```python
from build123d import *

# Parameters (mm, degrees)
SKETCH1_W                      = 88.6
SKETCH1_H                      = 58.4
BOSS_EXTRUDE1_DEPTH            = 1.6
F_2_7_2_7_DIAMETER_HOLE1_D     = 2.7
F_2_7_2_7_DIAMETER_HOLE1_DEPTH = 5.1
F_2_7_2_7_DIAMETER_HOLE1_TIP   = 0.811161836
LPATTERN1_COUNT                = 20
LPATTERN1_PITCH                = 2.54
LPATTERN1_COUNT_DIR2           = 2
LPATTERN1_PITCH_DIR2           = 2.54


with BuildPart() as part:
    # Sketch1 → Boss-Extrude1 (new body)
    with BuildSketch(Plane(origin=(0, 0, 0), x_dir=(1, 0, 0), z_dir=(0, 1, 0))):
        with Locations((11.8, 25.7)):
            Rectangle(SKETCH1_W, SKETCH1_H)
    extrude(amount=BOSS_EXTRUDE1_DEPTH)

    # Ø2.7 (2.7) Diameter Hole1
    with Locations(Plane(origin=(-29, 1.6, -49), x_dir=(0, 0, 1), z_dir=(0, 1, 0))):
        with Locations((0, 0), (0, 58), (49, 58), (49, 0)):
            Hole(F_2_7_2_7_DIAMETER_HOLE1_D / 2, depth=F_2_7_2_7_DIAMETER_HOLE1_DEPTH)
            with Locations((0, 0, -(F_2_7_2_7_DIAMETER_HOLE1_DEPTH + F_2_7_2_7_DIAMETER_HOLE1_TIP / 2))):  # 118° drill point
                Cone(0, F_2_7_2_7_DIAMETER_HOLE1_D / 2, F_2_7_2_7_DIAMETER_HOLE1_TIP, mode=Mode.SUBTRACT)

    # Sketch3 → Ø1.05 (1.05) Diameter Hole1 (revolve, cut)
    with BuildSketch(Plane(origin=(-24.13, 1.6, 1.27), x_dir=(0, 0, 1), z_dir=(1, 0, 0))):
        Polygon((0, 0), (0, 5.415451825), (0.525, 5.1), (0.525, 0), align=None)
    f_1_05_1_05_diameter_hole1 = revolve(axis=Axis((-24.13, 7.95, 1.27), (0, -1, 0)), mode=Mode.SUBTRACT)

    # LPattern1: 1.05 _1.05_ Diameter Hole1 20 × 2
    with Locations(*[(i * LPATTERN1_PITCH, 0, -j * LPATTERN1_PITCH_DIR2) for i in range(LPATTERN1_COUNT) for j in range(LPATTERN1_COUNT_DIR2) if (i, j) != (0, 0)]):
        add(f_1_05_1_05_diameter_hole1, mode=Mode.SUBTRACT)


solid = part.part
```
Work out the finished part from the listing and answer in its coordinate system (mm). Give positions to 0.01 mm unless a question says otherwise; leave off trailing zeros. Loops run counter-clockwise (first coordinate to the right, second up) from the corner with the lowest first, then second, coordinate; pieces in that order, holes last. Notation, with made-up numbers: M 38,40 L 49,40 A17 cw 49,47 Z; hole C 0.5,20 d3. An arc over 180 degrees is marked long. One line per item, written item: value. Start each with the question number.
1. Determine the mould class of faces 1 (the face through (-32.5, 1, -25)), 2 (the face through (11, 1, 3.5)), 3 (the face through (27.68, 0.79, 0.29)) for opening direction Z: released by +Z, released by -Z, zero draft, split by the parting line, or undercut.
2. This flat-tipped pin is pushed along its axis until it touches: P1, Ø0.8, axis at x = 16.51, z = -1.27, coming from the -Y side. Where does it stop, or does it pass through?
3. Find the intervals of material crossed by probe 1 along Z at (x, y) = (24.13, 0.7) (3 decimals); probe 2 along X at (y, z) = (1.15, -48), in increasing order.
4. Find section A-A (z = -49). Give the vertices of the cut face in (x, y).
Reported:
1. face 1: zero draft
1. face 2: released by +Z
1. face 3: undercut
2. P1: passes through
3. probe 1: z = -54.9 to -1.795, -0.745 to 0.745, 1.795 to 3.5
3. probe 2: x = -32.5 to -29.91, -28.09 to 28.09, 29.91 to 56.1
4. outline: M -32.5,0 L -30.35,0 L -30.35,1.6 L -32.5,1.6 Z; M -27.65,0 L 27.65,0 L 27.65,1.6 L -27.65,1.6 Z; M 30.35,0 L 56.1,0 L 56.1,1.6 L 30.35,1.6 Z
